Could you check a few things on this model? Use its own coordinates, in mm. Face numbers are marked on the shaded views. A direction names the side the tool comes from. Coordinates: 2 decimals unless noted, no trailing zeros. Loops run counter-clockwise (first coordinate to the right, second up) from the corner with the lowest first, then second, coordinate; pieces in that order, holes last.
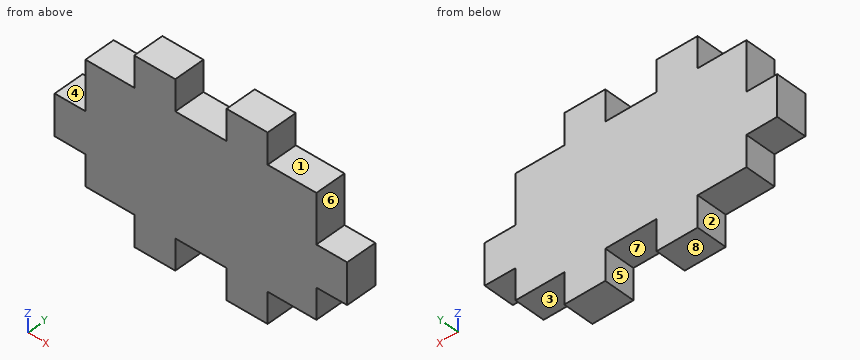
from build123d import *

# Parameters (mm, degrees)
SKETCH1_W           = 30
SKETCH1_H           = 50
BOSS_EXTRUDE1_DEPTH = 3
SKETCH2_W           = 7.75
SKETCH2_H           = 3
SKETCH2_W_2         = 5
CUT_EXTRUDE1_DEPTH  = 10
CUT_EXTRUDE2_DEPTH  = 10
SKETCH4_W           = 7.75
SKETCH4_H           = 3
SKETCH4_W_2         = 5
CUT_EXTRUDE3_DEPTH  = 10
CUT_EXTRUDE4_DEPTH  = 3


with BuildPart() as part:
    # Sketch1 → Boss-Extrude1 (new body)
    with BuildSketch(Plane(origin=(0, 0, 0), x_dir=(1, 0, 0), z_dir=(0, 1, 0))):
        Rectangle(SKETCH1_W, SKETCH1_H)
    extrude(amount=BOSS_EXTRUDE1_DEPTH)

    # Sketch2 → Cut-Extrude1 (cut)
    with BuildSketch(Plane(origin=(0, 3, 0), x_dir=(1, 0, 0), z_dir=(0, 1, 0))):
        with Locations((11.125, 23.5)):
            Rectangle(SKETCH2_W, SKETCH2_H)
        with Locations((0.75, 23.5)):
            Rectangle(SKETCH2_W_2, SKETCH2_H)
        with Locations((-9.625, 23.5)):
            Rectangle(SKETCH2_W, SKETCH2_H)
    extrude(amount=-CUT_EXTRUDE1_DEPTH, mode=Mode.SUBTRACT)

    # Sketch3 → Cut-Extrude2 (cut)
    with BuildSketch(Plane(origin=(0, 3, 0), x_dir=(1, 0, 0), z_dir=(0, 1, 0))):
        Polygon((-13.5, 22), (-13.5, 7.2), (33.838871071, 7.2), (23.912216497, -42.141377109), (-28.226414581, -62.151393572), (-28.226414581, 29.547983922), (-12.54526701, 26.393200971), align=None)
    extrude(amount=-CUT_EXTRUDE2_DEPTH, mode=Mode.SUBTRACT)

    # Sketch4 → Cut-Extrude3 (cut)
    with BuildSketch(Plane(origin=(0, 3, 0), x_dir=(1, 0, 0), z_dir=(0, 1, 0))):
        with Locations((11.125, 8.7)):
            Rectangle(SKETCH4_W, SKETCH4_H)
        with Locations((-9.625, 8.7)):
            Rectangle(SKETCH4_W, SKETCH4_H)
        with Locations((0.75, 8.7)):
            Rectangle(SKETCH4_W_2, SKETCH4_H)
    extrude(amount=-CUT_EXTRUDE3_DEPTH, mode=Mode.SUBTRACT)

    # Sketch5 → Cut-Extrude4 (cut)
    with BuildSketch(Plane(origin=(0, 3, 0), x_dir=(1, 0, 0), z_dir=(0, 1, 0))):
        Polygon((-10.5, 10.2), (-10.5, 15), (-13.5, 15), (-13.5, 18.977632451), (-10.5, 19), (-10.5, 22), (-14.44173644, 22), (-14.44173644, 10.2), align=None)
        Polygon((15.94173644, 22), (15.94173644, 10.2), (12, 10.2), (12, 15), (15, 15), (15, 18.977632451), (12, 19), (12, 22), align=None)
    extrude(amount=-CUT_EXTRUDE4_DEPTH, mode=Mode.SUBTRACT)


solid = part.part
(1) Imagine slicing it at C-C, the plane x = 8. Write out the boundary of the cut face in (y, z).
Answers:
outline: (0, -22) - (3, -22) - (3, -10.2) - (0, -10.2) - close
(2) We'd pull the mould along X, two halves only. Please class the marked faces 6, 7 and 8: +X half, -X half, draft (parallel to the pull), parting line (faces both ways), or undercut.
Answers:
face 6: +X half
face 7: undercut
face 8: draft
(3) Imagine slicing it at D-D, the plane z = -12.75. Write out the boundary of the cut face in (x, y).
Answers:
outline: (-10.5, 0) - (12, 0) - (12, 3) - (-10.5, 3) - close
(4) Which directions (+Z, -Z, +X, -X, +Y, -Y) give clear straight access to the entire face, cutting with the end or side of a thin tool? Please do the marked faces 1, 2, 3, 4 and 5.
Answers:
face 1: +Z, +X, +Y, -Y
face 2: -Z, -X, +Y, -Y
face 3: -Z, +X, +Y, -Y
face 4: +Z, -X, +Y, -Y
face 5: -Z, +Y, -Y
(5) Imagine slicing it at A-A, the plane z = -23. Write out the boundary of the cut face in (x, y).
Answers:
outline: (-5.75, 0) - (-1.75, 0) - (-1.75, 3) - (-5.75, 3) - close; (3.25, 0) - (7.25, 0) - (7.25, 3) - (3.25, 3) - close
(6) Imagine slicing it at B-B, the plane y = 2.6. Write out the boundary of the cut face in (x, z).
Answers:
outline: (-13.5, -18.98) - (-10.5, -19) - (-10.5, -22) - (-5.75, -22) - (-5.75, -25) - (-1.75, -25) - (-1.75, -22) - (3.25, -22) - (3.25, -25) - (7.25, -25) - (7.25, -22) - (12, -22) - (12, -19) - (15, -18.98) - (15, -15) - (12, -15) - (12, -10.2) - (7.25, -10.2) - (7.25, -7.2) - (3.25, -7.2) - (3.25, -10.2) - (-1.75, -10.2) - (-1.75, -7.2) - (-5.75, -7.2) - (-5.75, -10.2) - (-10.5, -10.2) - (-10.5, -15) - (-13.5, -15) - close
(7) For pin 1 (0.9 mm diameter, centred on y = 2, z = -23.5, fed in from -X); pin 2 (1.5 mm diameter, centred on y = 1.5, z = -24, fed in from +X); pin 3 (1.5 mm diameter, centred on y = 1.5, z = -21, fed in from +X), each with a flat end and sliding along its axis, tell me the tip position at first contact or that it passes through.
Answers:
pin 1: stops at x = -5.75
pin 2: stops at x = 7.25
pin 3: stops at x = 12
(8) I need wall thicknesses on probe 1 along X at (y, z) = (1.35, -8.75); probe 2 along Z at (x, y) = (1.5, 1); probe 3 along X at (y, z) = (2, -13). Which ranges of each line are inside material? Lowest first, please.
Answers:
probe 1: x = -5.75 to -1.75, 3.25 to 7.25
probe 2: z = -22 to -10.2
probe 3: x = -10.5 to 12
